Autodesk Inventor part; units mm, degrees
ref_plane "YZ Plane" through (0, 0, 0) normal (1, 0, 0) x (0, 1, 0)
ref_plane "XZ Plane" through (0, 0, 0) normal (0, 1, 0) x (-1, 0, 0)
ref_plane "XY Plane" through (0, 0, 0) normal (0, 0, 1) x (1, 0, 0)
sketch "Эскиз1" plane through (0, 0, 0) normal (0, 0, 1) x (1, 0, 0)
  line L0 (0, 0) -> (25.5, 0) construction
  line L1 (0, -3.5) -> (25.5, -3.5)
  line L2 (25.5, 3.5) -> (0, 3.5)
  arc A0 (0, 3.5) -> (0, -3.5) centre (0, 0) ccw
  arc A1 (25.5, -3.5) -> (25.5, 3.5) centre (25.5, 0) ccw
  point P0 (12.75, 0)
  dimension "d3" = 25.5
  dimension "d4" = 7
extrude "Выдавливание1" add sketch "Эскиз1" along normal blind 1.5
sketch "Эскиз2" plane through (0, 0, 1.5) normal (0, 0, 1) x (1, 0, 0)
  circle A0 centre (0, 0) radius 1.25
  dimension "d7" = 2.5
extrude "Выдавливание2" add sketch "Эскиз2" along normal blind 5
sketch "Эскиз4" plane through (0, 0, 1.5) normal (0, 0, 1) x (1, 0, 0)
  line L0 (0, -3.5) -> (25.5, -3.5) construction
  arc A0 (0, 3.5) -> (0, -3.5) centre (0, 0) ccw construction
  line L1 (25.5, 3.5) -> (0, 3.5) construction
  arc A1 (25.5, -3.5) -> (25.5, 3.5) centre (25.5, 0) ccw construction
  line L2 (25.5, -3.5) -> (14, -3.5)
  line L3 (14, 3.5) -> (25.5, 3.5)
  arc A2 (25.5, -3.5) -> (25.5, 3.5) centre (25.5, 0) ccw
  line L4 (14, 3.5) -> (14, -3.5)
  dimension "d15" = 11.5
extrude "Выдавливание4" add sketch "Эскиз4" along normal blind 2.9
sketch "Эскиз5" plane through (0, 0, 4.4) normal (0, 0, 1) x (1, 0, 0)
  circle A0 centre (26.5, 0) radius 0.5
  circle A1 centre (16.5, 0) radius 0.5
  line L0 (16.5, 0) -> (21.5, 0) construction
  line L1 (21.5, 0) -> (26.5, 0) construction
  arc A2 (25.5, -3.5) -> (25.5, 3.5) centre (25.5, 0) ccw construction
  point P0 (0, 0)
  point P1 (29, 0)
  dimension "d18" = 1
  dimension "d25" = 10
  dimension "d26" = 2.5
hole "Отверстие1" at (16.5, 0, 4.4) at (26.5, 0, 4.4) direction (0, 0, -1) diameter 1 end through all countersink diameter 1.5 countersink angle 90
properties part number "элемент-1"
Source: CAD feature listing. Evaluate the final solid. Frame: model axes, mm. A direction names the side the tool comes from. Give positions to 0.01 mm unless a question says otherwise; leave off trailing zeros. Loops run counter-clockwise (first coordinate to the right, second up) from the corner with the lowest first, then second, coordinate; pieces in that order, holes last. Notation, with made-up numbers: (58.5, 86) -> (70.5, 86) arc R9 ccw to (70.5, 102) -> close; hole circle Ø3 at (-21.5, -23.75). An arc over 180 degrees is marked (long way). Use a Markdown table: item, result. Add a question column.
1) Section query B-B, the plane x = 16.5. Return the cut outline in (y, z), then the cut area to 3 significant figures.
2) Reachability of faces 4 (the face through (16, -3.5, 2)), 5 (the face through (21, 0, 4.4)) from +Z, -Z, +X, -X, +Y, -Y: full face, straight path, thin tool, end or side. Return the list, or none.
3) Pull-direction query (Y, two-part tool) for faces 1 (the face through (-0.27, 1.22, 3.96)), 2 (the face through (14, 0, 3)), 3 (the face through (16, 0, 2)); classes: +Y half, -Y half, draft (parallel to the pull), parting line (faces both ways), or undercut.
4) Section query A-A, the plane z = 2.25. Return the cut outline in (x, y), then the cut area to 3 significant figures.
5) Section query C-C, the plane y = 0. Return the cut outline in (x, z).
6) Line query: line 1 along X through (y, z) = (0, 1.3); line 2 along Y through (x, z) = (16.5, 2.15); line 3 along Z through (x, y) = (-1, 3). Output: solid intervals per line, ascending. Write a range as [from, to].
7) First-contact query: pin 1 (1.5 mm diameter, centred on y = 1, z = 1, fed in from -X); pin 2 (1.5 mm diameter, centred on y = 1, z = 6, fed in from +X); pin 3 (3 mm diameter, centred on x = 23, y = -0.5, fed in from +Z). Flat tips, straight axial feed; report the tip coordinate or a pass-through.
8) Section query D-D, the plane z = 1. Return the cut outline in (x, y).
Numbers:
| question | item | result |
|---|---|---|
| 1 | outline | (-3.5, 0) -> (-0.5, 0) -> (-0.5, 4.15) -> (-0.75, 4.4) -> (-3.5, 4.4) -> close; (0.5, 0) -> (3.5, 0) -> (3.5, 4.4) -> (0.75, 4.4) -> (0.5, 4.15) -> close |
| 1 | area | 26.3 mm2 |
| 2 | face 4 | +Z, -Z, +X, -X, -Y |
| 2 | face 5 | +Z, +X, +Y, -Y |
| 3 | face 1 | parting line |
| 3 | face 2 | draft |
| 3 | face 3 | undercut |
| 4 | outline | circle Ø2.5 at (0, 0); (14, -3.5) -> (25.5, -3.5) arc R3.5 ccw to (25.5, 3.5) -> (14, 3.5) -> close; hole circle Ø1 at (16.5, 0); hole circle Ø1 at (26.5, 0) |
| 4 | area | 103 mm2 |
| 5 | outline | (-3.5, 0) -> (16, 0) -> (16, 4.15) -> (15.75, 4.4) -> (14, 4.4) -> (14, 1.5) -> (1.25, 1.5) -> (1.25, 6.5) -> (-1.25, 6.5) -> (-1.25, 1.5) -> (-3.5, 1.5) -> close; (17, 0) -> (26, 0) -> (26, 4.15) -> (25.75, 4.4) -> (17.25, 4.4) -> (17, 4.15) -> close; (27, 0) -> (29, 0) -> (29, 4.4) -> (27.25, 4.4) -> (27, 4.15) -> close |
| 6 | line 1 | x = [-3.5, 16], [17, 26], [27, 29] |
| 6 | line 2 | y = [-3.5, -0.5], [0.5, 3.5] |
| 6 | line 3 | z = [0, 1.5] |
| 7 | pin 1 | stops at x = -3.49 |
| 7 | pin 2 | stops at x = 1.22 |
| 7 | pin 3 | stops at z = 4.4 |
| 8 | outline | (0, -3.5) -> (25.5, -3.5) arc R3.5 ccw to (25.5, 3.5) -> (0, 3.5) arc R3.5 ccw to start; hole circle Ø1 at (16.5, 0); hole circle Ø1 at (26.5, 0) |
